Build history of the part. All positions in model axes, mm. Face numbers are marked on the shaded views. A direction names the side the tool comes from. Round coordinates to 2 decimals unless told otherwise and drop trailing zeros. Write each loop counter-clockwise with the first axis right and the second up, starting at its lowest first coordinate (ties: lowest second). Pieces come first, ordered by that corner, then holes. Notation, with made-up numbers: (65.25, 29.5) -> (114.25, 29.5) arc R9 cw to (114.25, 33.5) -> close; hole circle Ø5 at (23.25, 56). An arc over 180 degrees is marked (long way). Answer in a Markdown table with one row per item.
```python
from build123d import *

# Parameters (mm, degrees)
EXTRUDE1_DEPTH      = 2.54
SKETCH2_R           = 1.7018
EXTRUDE2_DEPTH      = 2.921
EXTRUDE5_DEPTH      = 2.032
SKETCH3_R           = 0.889
EXTRUDE3_DEPTH      = 4.953
EXTRUDE4_DEPTH      = 4.819904
CIRPATTERN1_COUNT   = 8
EXTRUDE13_DEPTH     = 4.819904
SKETCH7_R           = 0.3175
EXTRUDE6_DEPTH      = 11.651707
EXTRUDE10_DEPTH     = 2.54
EXTRUDE12_DEPTH     = 1.27
DRAFT5_ANGLE        = 1
DRAFT6_ANGLE        = 1
DRAFT7_ANGLE        = -0.5
FILLET1_R           = 0.254
CHAMFER1_SIZE       = 0.381
CHAMFER1_SIZE2      = 0.659911
EXTRUDE14_DEPTH     = 0.6604
BOSS_EXTRUDE1_DEPTH = 4.159504
CUT_EXTRUDE1_DEPTH  = 1.5
CHAMFER3_SIZE       = 0.1016
CHAMFER4_SIZE       = 0.3048


with BuildPart() as part:
    # Sketch1 → Extrude1 (new body)
    with BuildSketch(Plane.XY):
        with BuildLine():
            Line((-1.924985, 1.924985), (-3.048, 3.048))
            Line((-3.048, 3.048), (-6.001338, 3.048))
            ThreePointArc((-6.001338, 3.048), (-6.602226, 1.310331), (-6.710486, -0.525108))
            Line((-6.710486, -0.525108), (-1.963941, -3.265527))
            ThreePointArc((-1.963941, -3.265527), (-0.983782, -3.671523), (0.068059, -3.81))
            Line((0.068059, -3.81), (4.259709, -3.81))
            ThreePointArc((4.259709, -3.81), (4.60741, -3.381272), (4.912126, -2.921))
            Line((4.912126, -2.921), (3.99071, -2.373079))
            ThreePointArc((3.99071, -2.373079), (3.640517, -1.933065), (3.66974, -1.371466))
            ThreePointArc((3.66974, -1.371466), (3.67694, 2.904446), (0.541494, 5.811758))
            ThreePointArc((0.541494, 5.811758), (0.285086, 5.809719), (0.088038, 5.645641))
            Line((0.088038, 5.645641), (-0.535349, 4.589543))
            Line((-0.535349, 4.589543), (0.837366, 2.953604))
            ThreePointArc((0.837366, 2.953604), (0.944247, 2.141765), (0.25364, 1.7018))
            Line((0.25364, 1.7018), (-1.386169, 1.7018))
            ThreePointArc((-1.386169, 1.7018), (-1.677774, 1.759804), (-1.924985, 1.924985))
        make_face()
    extrude(amount=EXTRUDE1_DEPTH)

    # Sketch2 → Extrude2 (add)
    with BuildSketch(Plane.XY.offset(2.54)):
        with Locations(Location((0, 0, 0), (0, 0, 90))):
            Circle(SKETCH2_R)
    extrude(amount=EXTRUDE2_DEPTH)

    # Sketch6 → Extrude5 (add)
    with BuildSketch(Plane.XY.offset(2.54)):
        with BuildLine():
            Line((0, 1.7018), (3.103645, 1.7018))
            ThreePointArc((3.103645, 1.7018), (3.829425, 1.396785), (4.119429, 0.664878))
            ThreePointArc((4.119429, 0.664878), (4.031669, -0.195019), (3.806175, -1.029451))
            ThreePointArc((3.806175, -1.029451), (3.434483, -1.516885), (2.850058, -1.7018))
            Line((2.850058, -1.7018), (0, -1.7018))
            ThreePointArc((0, -1.7018), (1.7018, 0), (0, 1.7018))
        make_face()
    extrude(amount=EXTRUDE5_DEPTH)

    # Sketch3 → Extrude3 (add)
    with BuildSketch(Plane.XY.offset(5.461)):
        Circle(SKETCH3_R)
    extrude(amount=EXTRUDE3_DEPTH)

    # Sketch4 → Extrude4 (cut)
    with BuildSketch(Plane(origin=(0, 0, 0), x_dir=(-1, 0, 0), z_dir=(0, 0, -1))):
        with BuildLine():
            Line((0, 0), (-0.311045, 0.750929))
            ThreePointArc((-0.311045, 0.750929), (-0.238333, 0.777072), (-0.163468, 0.796192))
            ThreePointArc((-0.163468, 0.796192), (0, 0.7366), (0.163468, 0.796192))
            ThreePointArc((0.163468, 0.796192), (0.238333, 0.777072), (0.311045, 0.750929))
            Line((0.311045, 0.750929), (0, 0))
        make_face()
    extrude4 = extrude(amount=-EXTRUDE4_DEPTH, mode=Mode.SUBTRACT)

    # CirPattern1: Extrude4 ×8 about axis
    cirpattern1_axis = Axis((0, 0, 0), (0, 0, 1))
    for i in range(1, CIRPATTERN1_COUNT):
        add(extrude4.rotate(cirpattern1_axis, i * 360 / CIRPATTERN1_COUNT), mode=Mode.SUBTRACT)

    # Sketch14 → Extrude13 (add)
    with BuildSketch(Plane(origin=(0, 0, 0), x_dir=(-1, 0, 0), z_dir=(0, 0, -1))):
        with BuildLine():
            Line((-0.730885, 0.3556), (0.730885, 0.3556))
            ThreePointArc((0.730885, 0.3556), (0, 0.8128), (-0.730885, 0.3556))
        make_face()
    extrude(amount=-EXTRUDE13_DEPTH)

    # Sketch7 → Extrude6 (cut, through all)
    with BuildSketch(Plane.XY.offset(4.572)):
        with Locations((3.019144, 0.144507)):
            Circle(SKETCH7_R)
    extrude(amount=-EXTRUDE6_DEPTH, mode=Mode.SUBTRACT)

    # Sketch11 → Extrude10 (cut)
    with BuildSketch(Plane(origin=(0, 0, 0), x_dir=(-1, 0, 0), z_dir=(0, 0, -1))):
        with BuildLine():
            ThreePointArc((-2.983619, -0.648448), (-2.234049, 0.261404), (-3.216173, 0.913414))
            ThreePointArc((-3.216173, 0.913414), (-3.503818, 0.716068), (-3.59637, 0.379737))
            ThreePointArc((-3.59637, 0.379737), (-3.559938, 0.063985), (-3.502801, -0.248683))
            ThreePointArc((-3.502801, -0.248683), (-3.316279, -0.543462), (-2.983619, -0.648448))
        make_face()
    extrude(amount=-EXTRUDE10_DEPTH, mode=Mode.SUBTRACT)

    # Sketch13 → Extrude12 (cut)
    with BuildSketch(Plane(origin=(0, 0, 0), x_dir=(-1, 0, 0), z_dir=(0, 0, -1))):
        with BuildLine():
            Line((2.93074, -1.240876), (5.181827, 0.05879))
            ThreePointArc((5.181827, 0.05879), (5.380013, 0.267231), (5.433245, 0.549882))
            ThreePointArc((5.433245, 0.549882), (5.372687, 0.978137), (5.278428, 1.400256))
            ThreePointArc((5.278428, 1.400256), (5.097164, 1.672638), (4.787412, 1.778))
            Line((4.787412, 1.778), (3.784472, 1.778))
            ThreePointArc((3.784472, 1.778), (3.590069, 1.739331), (3.425261, 1.62921))
            Line((3.425261, 1.62921), (2.82301, 1.026959))
            ThreePointArc((2.82301, 1.026959), (2.666482, 0.885883), (2.496186, 0.761776))
            ThreePointArc((2.496186, 0.761776), (2.313241, 0.550864), (2.269383, 0.27513))
            ThreePointArc((2.269383, 0.27513), (2.277738, -0.194184), (2.19006, -0.65531))
            ThreePointArc((2.19006, -0.65531), (2.36169, -1.199441), (2.93074, -1.240876))
        make_face()
    extrude(amount=-EXTRUDE12_DEPTH, mode=Mode.SUBTRACT)

    # Draft5
    draft5_faces = [part.faces().sort_by_distance(p)[0] for p in [
        (3.316279, -0.543462, 1.27),
        (3.559938, 0.063985, 1.27),
        (3.503818, 0.716068, 1.27),
        (2.234049, 0.261404, 1.27),
    ]]
    draft(draft5_faces, Plane(origin=(0.896458, 0.316881, 2.54), x_dir=(-1, 0, 0), z_dir=(0, 0, -1)), DRAFT5_ANGLE)

    # Draft6
    draft6_faces = [part.faces().sort_by_distance(p)[0] for p in [
        (-2.666482, 0.885883, 0.635),
        (-2.313241, 0.550864, 0.635),
        (-2.277738, -0.194184, 0.635),
        (-2.36169, -1.199441, 0.635),
        (-4.056284, -0.591043, 0.635),
        (-5.380013, 0.267231, 0.635),
        (-5.372687, 0.978137, 0.635),
        (-5.097164, 1.672638, 0.635),
        (-4.285942, 1.778, 0.635),
        (-3.590069, 1.739331, 0.635),
        (-3.124136, 1.328085, 0.635),
    ]]
    draft(draft6_faces, Plane(origin=(0, 0, 1.27), x_dir=(-1, 0, 0), z_dir=(0, 0, -1)), DRAFT6_ANGLE)

    # Draft7
    draft7_faces = [part.faces().sort_by_distance(p)[0] for p in [
        (-0.889, 0, 7.9375),
        (0, -1.7018, 4.0005),
        (1.425029, -1.7018, 3.556),
        (4.60741, -3.381272, 1.27),
        (2.163884, -3.81, 1.27),
        (-0.983782, -3.671523, 1.27),
        (-4.337213, -1.895318, 1.27),
        (-6.602226, 1.310331, 1.27),
        (-4.524669, 3.048, 1.27),
        (-2.486492, 2.486492, 1.27),
        (-1.677774, 1.759804, 1.27),
        (0.285086, 5.809719, 1.27),
        (-0.223656, 5.117592, 1.27),
        (0.151008, 3.771574, 1.27),
        (0.944247, 2.141765, 1.27),
        (0.709356, 1.7018, 2.646746),
        (3.829425, 1.396785, 3.556),
        (3.434483, -1.516885, 3.556),
        (4.451418, -2.647039, 1.27),
        (3.640517, -1.933065, 1.27),
        (3.67694, 2.904446, 2.286),
    ]]
    draft(draft7_faces, Plane(origin=(0, 0, 0), x_dir=(-1, 0, 0), z_dir=(0, 0, -1)), DRAFT7_ANGLE)

    # Fillet1
    fillet1_edges = [part.edges().sort_by_distance(p)[0] for p in [
        (-0.841343, 0, 5.461),
    ]]
    fillet(fillet1_edges, radius=FILLET1_R)

    # Chamfer1
    chamfer1_edges = [part.edges().sort_by_distance(p)[0] for p in [
        (0, 0.3556, 0),
    ]]
    chamfer1_side = [part.faces().sort_by_distance(p)[0] for p in [
        (0.337088, 5.667766, 0),
    ]]
    chamfer(chamfer1_edges, length=CHAMFER1_SIZE, length2=CHAMFER1_SIZE2, reference=chamfer1_side[0])

    # Sketch16 → Extrude14 (cut)
    with BuildSketch(Plane(origin=(0, 0, 0), x_dir=(-1, 0, 0), z_dir=(0, 0, -1))):
        with BuildLine():
            Line((0.730885, 0.3556), (-0.730885, 0.3556))
            ThreePointArc((-0.730885, 0.3556), (0, -0.8128), (0.730885, 0.3556))
        make_face()
    extrude(amount=-EXTRUDE14_DEPTH, mode=Mode.SUBTRACT)

    # Sketch17 → Boss-Extrude1 (add)
    with BuildSketch(Plane(origin=(0, 0, 0.6604), x_dir=(-1, 0, 0), z_dir=(0, 0, -1))):
        with BuildLine():
            Line((0.730885, 0.3556), (0.64508, 0.3556))
            ThreePointArc((0.64508, 0.3556), (0, -0.7366), (-0.64508, 0.3556))
            Line((-0.64508, 0.3556), (-0.730885, 0.3556))
            ThreePointArc((-0.730885, 0.3556), (0, -0.8128), (0.730885, 0.3556))
        make_face()
    extrude(amount=-BOSS_EXTRUDE1_DEPTH)

    # Sketch18 → Cut-Extrude1 (cut)
    with BuildSketch(Plane(origin=(0, 0, 0), x_dir=(-1, 0, 0), z_dir=(0, 0, -1))):
        with BuildLine():
            Line((0.730885, 0.3556), (-0.730885, 0.3556))
            ThreePointArc((-0.730885, 0.3556), (0, -0.8128), (0.730885, 0.3556))
        make_face()
    extrude(amount=-CUT_EXTRUDE1_DEPTH, mode=Mode.SUBTRACT)

    # Chamfer3
    # the kernel refuses this chamfer: 0.1016 mm, written as the material it takes off along each edge
    with BuildSketch(Plane(origin=(0, 0, 1.5), x_dir=(0.6528066394182584, 0.7575245814700933, 0), z_dir=(-0.7575245814700933, 0.6528066394182584, 0))) as chamfer3_piece_1_section:
        Polygon((0.7366, -CHAMFER3_SIZE), (0.7366 + CHAMFER3_SIZE, 0), (0.7366, 0), align=None)
    chamfer3_piece_1 = revolve(axis=Axis((0, 0, 1.5), (0, 0, -1)), revolution_arc=278.492908, mode=Mode.PRIVATE)
    chamfer3_piece_1 = split(chamfer3_piece_1, bisect_by=Plane(origin=(0, 0.3556, 1.563136), z_dir=(0, -1, 0)), keep=Keep.TOP, mode=Mode.PRIVATE)
    chamfer3_piece_1 = chamfer3_piece_1 & Plane(origin=(0, 0, 1.563136), x_dir=(0.9795673076923074, 0.20111660722189145, 0), z_dir=(0, 0, -1)) * Cylinder(0.8128, 4, mode=Mode.PRIVATE)
    add(chamfer3_piece_1, mode=Mode.SUBTRACT)

    # Chamfer4
    chamfer4_edges = [part.edges().sort_by_distance(p)[0] for p in [
        (0, -0.8128, 0),
    ]]
    chamfer(chamfer4_edges, length=CHAMFER4_SIZE)


solid = part.part
```
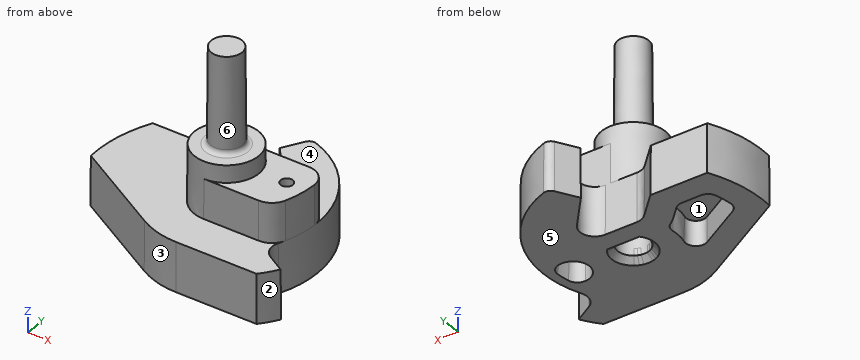
Q1. Wall check: line 1 (X direction, y = 0, z = 4.25); line 2 (X direction, y = 0, z = 0.65); line 3 (Z direction, x = -4.75, y = -0.75). Give the ranges that are in metal, low to high. Write a range as [from, to].
A:
| item | result |
|---|---|
| line 1 | [-1.66, -0.74], [0.74, 2.74], [3.3, 4.03] |
| line 2 | [-6.73, -5.1], [-2.28, -0.81], [0.81, 2.21], [3.58, 4.06] |
| line 3 | [0, 2.54] |
Q2. Saw through at B-B on x = -4. Write the cut outline in (y, z).
A:
| item | result |
|---|---|
| outline | (-2.09, 0) -> (-0.65, 0) -> (-0.62, 1.27) -> (1.78, 1.27) -> (1.8, 0) -> (3.05, 0) -> (3.03, 2.54) -> (-2.06, 2.54) -> close |
Q3. Saw through at D-D on z = 7.5. Write the cut outline in (x, y), plus the area to 3 significant figures.
A:
| item | result |
|---|---|
| outline | circle Ø1.65 at (0, 0) |
| area | 2.13 mm² |
Q4. Drop flat-ended pins along their axis: P1, Ø2, axis at x = -4, y = 1.5, coming from the +Z side; P2, Ø5.5, axis at x = -2, y = -0.5, coming from the +Z side; P3, Ø4, axis at x = 1.5, z = 5, coming from the -Y side; P4, Ø3.5, axis at x = 3, y = 0.5, coming from the +Z side. Give the stop position or say it passes through.
A:
| item | result |
|---|---|
| P1 | z = 2.54 |
| P2 | z = 10.41 |
| P3 | y = -1.68 |
| P4 | z = 5.46 |
Q5. Saw through at A-A on z = 1.75. Write the cut outline in (x, y).
A:
| item | result |
|---|---|
| outline | (-6.7, -0.52) -> (-1.96, -3.25) arc R4.05 ccw to (0.07, -3.79) -> (4.25, -3.79) arc R5.7 ccw to (4.89, -2.93) -> (3.98, -2.39) arc R0.81 cw to (3.66, -1.37) arc R5.32 ccw to (0.54, 5.8) arc R0.37 ccw to (0.1, 5.64) -> (-0.52, 4.59) -> (0.85, 2.96) arc R0.78 cw to (0.25, 1.69) -> (-1.39, 1.69) arc R0.78 cw to (-1.94, 1.91) -> (-3.05, 3.03) -> (-5.99, 3.03) arc R6.72 ccw to start; hole (-0.65, 0.36) arc R0.74 ccw (long way) to (0.65, 0.36) -> close; hole (2.98, -0.66) arc R0.52 ccw to (3.52, -0.25) arc R4.84 ccw to (3.61, 0.38) arc R0.52 ccw to (3.22, 0.93) arc R0.81 ccw (long way) to start |
Q6. Which spindle directions (+Z, -Z, +X, -X, +Y, -Y) get a long thin tool onto all of the face, cutting with end or side? Do the marked faces 5 and 6. Say none if no direction does.
A:
| item | result |
|---|---|
| face 5 | -Z, +X, -X, +Y, -Y |
| face 6 | +Z |
Q7. Two-plate mould, pull along X, no slides. Class the marked faces 1, 2, 3 and 4: released by +X, released by -X, zero draft, split by the parting line, or undercut.
A:
| item | result |
|---|---|
| face 1 | undercut |
| face 2 | released by +X |
| face 3 | released by -X |
| face 4 | zero draft |
Q8. Saw through at C-C on z = 3. Write the cut outline in (x, y) (1 decimal), plus the area to 3 significant figures.
A:
| item | result |
|---|---|
| outline | (0, -1.7) -> (2.9, -1.7) arc R1 ccw to (3.8, -1) arc R5.3 ccw to (4.1, 0.7) arc R1 ccw to (3.1, 1.7) -> (0, 1.7) arc R1.7 ccw to start; hole (-0.6, 0.4) arc R0.7 ccw (long way) to (0.6, 0.4) -> close; hole circle Ø0.6 at (3, 0.1) |
| area | 15.7 mm² |
